The listing builds one solid part. Answer for the finished solid, in the listing's coordinates (mm). Round coordinates to 2 decimals unless told otherwise and drop trailing zeros. Order: outer loops, then holes, each group sorted by start corner. A loop starts at its lowest first (then second) coordinate and runs counter-clockwise, first axis right, second up. Notation, with made-up numbers: (32.25, -21.75) - (71.25, -21.75) arc R30 cw to (71.25, 13.25) - close; hole circle Ø8 at (-11, 76). An arc over 180 degrees is marked (long way). Use CSV: the item, a comma, the result in double quotes. Start each with the question number.
Item 1: Find section C-C, the plane y = 48. Give the vertices of the cut face in (x, z).
Item 2: Find section A-A, the plane z = 7. Give the vertices of the cut face in (x, y), plus the area to 3 significant figures.
Item 3: Straight lines are drawn through the part: line 1 along X through (y, z) = (8, 1.5); line 2 along X through (y, z) = (16.5, 7.25); line 3 along Y through (x, z) = (-52.5, 9.5). For each, find the intervals that lie inside material, in ascending order. Write a range as [from, to].
Item 4: Find section B-B, the plane x = 113. Give the vertices of the cut face in (y, z).
Item 5: Flat-ended cylindrical pins translate along their axes: P1, Ø1, axis at y = 49, z = 7, coming from the -X side; P2, Ø6, axis at x = -41, z = 3.5, coming from the -Y side; P3, Ø3, axis at y = 56.5, z = 7, coming from the -X side. Find the tip coordinate at first contact, or state that the pin passes through.
Item 6: Determine the mould class of faces 1 (the flat face through (-98.41, 49.1, 4.93)), 2 (the cylindrical face through (-147.68, 7.27, 5.07)), 3 (the cylindrical face through (-126.01, 13.31, 4.93)) for opening direction Y: +Y half, -Y half, draft (parallel to the pull), parting line (faces both ways), or undercut.
Item 7: Find section D-D, the plane x = -116. Give the vertices of the cut face in (y, z), plus the area to 3 significant figures.
```python
from build123d import *

# Parameters (mm, degrees)
SKETCH2_R           = 7.5
BOSS_EXTRUDE1_DEPTH = 10
FILLET1_R           = 15
FILLET2_R           = 15
FILLET3_R           = 15


with BuildPart() as part:
    # Sketch2 → Boss-Extrude1 (new body)
    with BuildSketch(Plane.XY):
        Polygon((-188.967985521, -4.587781845), (-49.180964379, 78.282699744), (217.267895037, 0.098297427), align=None)
        with Locations((-133.163966534, 11.056935849)):
            Circle(SKETCH2_R, mode=Mode.SUBTRACT)
        with Locations((-47.143917344, 62.052535044)):
            Circle(SKETCH2_R, mode=Mode.SUBTRACT)
        with Locations((116.819402044, 13.94058532)):
            Circle(SKETCH2_R, mode=Mode.SUBTRACT)
    extrude(amount=BOSS_EXTRUDE1_DEPTH)

    # Fillet1
    fillet1_edges = [part.edges().sort_by_distance(p)[0] for p in [
        (217.267895037, 0.098297427, 5),
    ]]
    fillet(fillet1_edges, radius=FILLET1_R)

    # Fillet2
    fillet2_edges = [part.edges().sort_by_distance(p)[0] for p in [
        (-49.180964379, 78.282699744, 5),
    ]]
    fillet(fillet2_edges, radius=FILLET2_R)

    # Fillet3
    fillet3_edges = [part.edges().sort_by_distance(p)[0] for p in [
        (-188.967985521, -4.587781845, 5),
    ]]
    fillet(fillet3_edges, radius=FILLET3_R)


solid = part.part
```
Worked out:
1,outline,"(-100.26, 0) - (54.02, 0) - (54.02, 10) - (-100.26, 10) - close"
2,outline,"(-140.81, 23.96) arc R15 ccw to (-132.99, -3.94) - (116.99, -1.06) arc R15 ccw to (121.04, 28.33) - (-42.92, 76.45) arc R15 ccw to (-54.79, 74.96) - close; hole circle Ø15 at (-133.16, 11.06); hole circle Ø15 at (-47.14, 62.05); hole circle Ø15 at (116.82, 13.94)"
2,area,"14,200 mm²"
3,line 1,"x = [-147.85, -140.01], [-126.32, 112.24], [121.4, 130.59]"
3,line 2,"x = [-147.14, -138.32], [-128, 109.77], [123.87, 131.6]"
3,line 3,"y = [-3.01, 56.8], [67.3, 76.06]"
4,outline,"(-1.1, 0) - (7.49, 0) - (7.49, 10) - (-1.1, 10) - close; (20.4, 0) - (30.69, 0) - (30.69, 10) - (20.4, 10) - close"
5,P1,"stops at x = -99.42"
5,P2,"stops at y = -2.92"
5,P3,"stops at x = -88.45"
6,face 1,"+Y half"
6,face 2,"parting line"
6,face 3,"undercut"
7,outline,"(-3.75, 0) - (38.67, 0) - (38.67, 10) - (-3.75, 10) - close"
7,area,"424 mm²"
